Check sheet for the modelled part. Datum: model origin and axes. Units: mm. Give positions to 0.01 mm unless a question says otherwise; leave off trailing zeros. Write each loop counter-clockwise with the first axis right and the second up, starting at its lowest first coordinate (ties: lowest second). Pieces come first, ordered by that corner, then holes. Notation, with made-up numbers: (72, -33) -> (109, -33) arc R23 cw to (109, -18) -> close; hole circle Ø7 at (0.25, 75.25). An arc over 180 degrees is marked (long way). Write each question's results on one line, items separated by ' | '. Start each with the question number.
```python
from build123d import *

# Parameters (mm, degrees)
BASE_FLANGE1_DEPTH = 3
HEM1_START         = -185.00035483
HEM1_DEPTH         = 297
HEM1_2_DEPTH       = 297


# Read off the part's stored shape, not the designer's step: Hem1
# Sheet-metal steps are written as plain solids
with BuildPart() as part:
    # Sketch1 → Base-Flange1 (new body)
    with BuildSketch(Plane.XY):
        Polygon((18.49964517, -243.314393939), (104.99964517, -243.314393939), (104.99964517, -108.314393939), (111.99964517, -108.314393939), (111.99964517, -102.314393939), (-185.00035483, -102.314393939), (-185.00035483, -108.314393939), (-178.00035483, -108.314393939), (-178.00035483, -243.314393939), (-91.50035483, -243.314393939), (-91.50035483, -263.314393939), (18.49964517, -263.314393939), align=None)
    extrude(amount=-BASE_FLANGE1_DEPTH)

    # Hem1 outline → Hem1 (cut)
    with BuildSketch(Plane.YZ.offset(HEM1_START)):
        with BuildLine():
            Line((-102.314393939, 0), (-102.441410593, 0))
            ThreePointArc((-102.441410593, 0), (-103.864904196, -2.16227766), (-106.314393939, -3))
            Line((-106.314393939, -3), (-102.314393939, -3))
            Line((-102.314393939, -3), (-102.314393939, 0))
        make_face()
    extrude(amount=HEM1_DEPTH, mode=Mode.SUBTRACT)

    # Hem1 2 outline → Hem1 2 (add)
    with BuildSketch(Plane.YZ.offset(HEM1_START)):
        with BuildLine():
            Line((-110.314393939, 1), (-107.314393939, 1))
            ThreePointArc((-107.314393939, 1), (-105.607287158, 1.707106781), (-106.314393939, 0))
            Line((-106.314393939, 0), (-102.441410593, 0))
            ThreePointArc((-102.441410593, 0), (-105.810376769, 4.968118785), (-110.314393939, 1))
        make_face()
    extrude(amount=HEM1_2_DEPTH)


solid = part.part
```
Item 1: Section check A-A on x = -158. Record the boundary of the cut face in (y, z), then the cut area to 3 significant figures.
Item 2: Section check B-B on z = -1.75. Record the boundary of the cut face in (x, y), then the cut area to 3 significant figures.
Item 3: Section check C-C on y = -216.5. Record the boundary of the cut face in (x, z), then the cut area to 3 significant figures.
Item 4: Section check D-D on x = -25. Record the boundary of the cut face in (y, z), then the cut area to 3 significant figures.
Item 5: Depth check by flat-ended pin: pin 1 Ø3.5 at (x, z) = (108.5, -2) entering from -Y; pin 2 Ø0.9 at (x, z) = (81.5, -2) entering from -Y; pin 3 Ø1.5 at (y, z) = (-252, -1) entering from -X. Enter the tip coordinate at first touch or a pass-through.
Item 6: Thickness scan on probe 1 along Z at (x, y) = (-91.5, -182.5); probe 2 along X at (y, z) = (-172.5, -1.5); probe 3 along Y at (x, z) = (70.5, -0.5). Record the ranges inside material, lowest first. Write a range as from..to.
Check sheet entries:
1) outline: (-243.31, -3) -> (-106.31, -3) arc R4 ccw (long way) to (-110.31, 1) -> (-107.31, 1) arc R1 cw (long way) to (-106.31, 0) -> (-243.31, 0) -> close | area: 446 mm^2
2) outline: (-185, -108.31) -> (-178, -108.31) -> (-178, -243.31) -> (-91.5, -243.31) -> (-91.5, -263.31) -> (18.5, -263.31) -> (18.5, -243.31) -> (105, -243.31) -> (105, -108.31) -> (112, -108.31) -> (112, -103.41) -> (-185, -103.41) -> close | area: 41,900 mm^2
3) outline: (-178, -3) -> (105, -3) -> (105, 0) -> (-178, 0) -> close | area: 849 mm^2
4) outline: (-263.31, -3) -> (-106.31, -3) arc R4 ccw (long way) to (-110.31, 1) -> (-107.31, 1) arc R1 cw (long way) to (-106.31, 0) -> (-263.31, 0) -> close | area: 506 mm^2
5) pin 1: stops at y = -108.31 | pin 2: stops at y = -243.31 | pin 3: stops at x = -91.5
6) probe 1: z = -3..0 | probe 2: x = -178..105 | probe 3: y = -243.31..-102.61
